Autodesk Inventor part; units mm, degrees
ref_plane "YZ Plane" through (0, 0, 0) normal (1, 0, 0) x (0, 1, 0)
ref_plane "XZ Plane" through (0, 0, 0) normal (0, 1, 0) x (-1, 0, 0)
ref_plane "XY Plane" through (0, 0, 0) normal (0, 0, 1) x (1, 0, 0)
sketch "スケッチ1" plane through (0, 0, 0) normal (0, 1, 0) x (-1, 0, 0)
  line L0 (75, 0) -> (105, -51.9615)
  line L1 (-75, 0) -> (-105, -51.9615)
  line L2 (0, -218.2384) -> (0, 36.3731)
  line L3 (147, 0) -> (-147, 0)
  line L4 (105, -51.9615) -> (30, -181.8653)
  line L5 (30, -181.8653) -> (-30, -181.8653)
  line L6 (-30, -181.8653) -> (-105, -51.9615)
  line L7 (75, 0) -> (-75, 0)
  line L8 (34, 0) -> (34, -24.3509)
  line L9 (34, -24.3509) -> (48.7058, -49.822)
  line L10 (48.7058, -49.822) -> (90, -25.9808)
  line L11 (45, 0) -> (45, -18) construction
  line L12 (45, -18) -> (34, -24.3509) construction
  line L13 (84.5, -87.4686) -> (63.4115, -75.2931)
  line L14 (63.4115, -75.2931) -> (48.7058, -49.822)
  line L15 (-34, 0) -> (-34, -24.3509)
  line L16 (-34, -24.3509) -> (-48.7058, -49.822)
  line L17 (-63.4115, -75.2931) -> (-48.7058, -49.822)
  line L18 (-84.5, -87.4686) -> (-63.4115, -75.2931)
  circle A0 centre (30, -32.75) radius 1.6
  circle A1 centre (-30, -32.75) radius 1.6
  line L19 (35.5295, -27) -> (-35.5295, -27)
  point P0 (0, 0)
  point P1 (0, 0)
  point P2 (0, -27)
  dimension "d1" = 150
  dimension "d2" = 60
  dimension "d3" = 60
  dimension "d6" = 60
  dimension "d30" = 60
  dimension "d31" = 18
  dimension "d32" = 30
  dimension "d33" = 41
  dimension "d34" = 3.2
  dimension "d35" = 30
  dimension "d36" = 32.75
  dimension "d37" = 27
extrude "プレート1" add sketch "スケッチ1" along normal blind 1.5 contours L14 L13 L4 L5 L2 L19 L9 | L2 L5 L6 L18 L17 L16 L19
sketch "スケッチ4" plane through (0, 1.5, 0) normal (0, 1, 0) x (1, 0, 0)
  circle A0 centre (30, 67.8013) radius 1.6
  circle A1 centre (45, 67.8013) radius 1.6
  line L0 (0, 218.2384) -> (0, -36.3731)
  circle A2 centre (-30, 67.8013) radius 1.6
  circle A3 centre (-45, 67.8013) radius 1.6
  line L1 (61.6173, 73.1025) -> (25, 73.1025)
  line L2 (25, 73.1025) -> (25, 62.5)
  line L3 (-61.6173, 73.1025) -> (-25, 73.1025)
  line L4 (-25, 73.1025) -> (-25, 62.5)
  line L5 (-25, 62.5) -> (25, 62.5)
  line L6 (-30, 73.1025) -> (30, 73.1025)
  line L7 (30, 73.1025) -> (30, 181.8653)
  line L8 (30, 181.8653) -> (-30, 181.8653)
  line L9 (-30, 181.8653) -> (-30, 73.1025)
  line L10 (-25, 62.5) -> (25, 62.5)
  line L11 (25, 62.5) -> (25, 73.1025)
  line L12 (25, 73.1025) -> (-25, 73.1025)
  line L13 (-25, 73.1025) -> (-25, 62.5)
  line L14 (30, 181.8653) -> (84.5, 87.4686)
  line L15 (76.75, 100.892) -> (30, 73.9008)
  line L16 (-30, 73.9008) -> (-76.75, 100.892)
  line L17 (-84.5, 87.4686) -> (-30, 181.8653)
  line L18 (84.5, 87.4686) -> (63.4115, 75.2931)
  line L19 (-63.4115, 75.2931) -> (-84.5, 87.4686)
  line L20 (-35.5295, 27) -> (-63.4115, 75.2931)
  line L21 (62.8673, 70.9375) -> (54.6673, 85.1403)
  arc A4 (54.6673, 85.1403) -> (44.275, 79.1403) centre (49.4712, 82.1403) ccw
  line L22 (44.275, 79.1403) -> (52.475, 64.9375)
  line L23 (52.475, 64.9375) -> (62.8673, 70.9375)
  line L24 (51.2321, 85.1903) -> (52.993, 82.1403)
  line L25 (52.993, 82.1403) -> (51.2321, 79.0903)
  line L26 (51.2321, 79.0903) -> (47.7102, 79.0903)
  line L27 (47.7102, 79.0903) -> (45.9493, 82.1403)
  line L28 (45.9493, 82.1403) -> (47.7102, 85.1903)
  line L29 (47.7102, 85.1903) -> (51.2321, 85.1903)
  point P0 (0, 0)
extrude "切り取り3" cut sketch "スケッチ4" against normal blind 1.5 contours A0 | A1 | L8 L7 L1 L6 L0 | L0 L6 L3 L9 L8 | L6 L2 L5 L0 | L0 L5 L4 L6 | L14 L15 A4 L7 | L9 L16 L17 | A4 L15 L29 L28 | L28 L29 L15 | A2 | A3
sketch "スケッチ5" plane through (0, 1.5, 0) normal (0, 1, 0) x (1, 0, 0)
  line L0 (-75, 44) -> (75, 44)
  circle A0 centre (-20, 41) radius 3
  circle A1 centre (20, 41) radius 3
  line L1 (-25, 62.5) -> (25, 62.5)
  line L2 (0, 62.5) -> (0, 27)
  line L3 (35.5295, 27) -> (-35.5295, 27)
  circle A2 centre (-20, 41) radius 1.6
  circle A3 centre (20, 41) radius 1.6
  circle A4 centre (0, 34) radius 1.6
  point P0 (0, 0)
  dimension "d41" = 6
  dimension "d42" = 6
  dimension "d43" = 40
  dimension "d44" = 3.2
  dimension "d45" = 3.2
  dimension "d46" = 3.2
  dimension "d47" = 7
extrude "切り取り4" cut sketch "スケッチ5" against normal blind 1.5 contours A4 L2 | L2 A4 | A2 | A3
sketch "スケッチ6" plane through (0, 1.5, 0) normal (0, 1, 0) x (1, 0, 0)
  ellipse E0 centre (-73.3666, 93.1522) end of major axis (-72.2841, 92.5272) minor radius 1.2133
  circle A0 centre (-48.4391, 79.9279) radius 1.6
  circle A1 centre (-73.3666, 93.1522) radius 1.6
  line L0 (0, 0) -> (0, 20.4537)
  circle A2 centre (48.4391, 79.9279) radius 1.6
  circle A3 centre (73.3666, 93.1522) radius 1.6
  circle A4 centre (-48.4391, 79.9279) radius 1.35
  dimension "d51" = 3.2
  dimension "d52" = 3.2
extrude "切り取り5" cut sketch "スケッチ6" against normal blind 1.5 contours E0 | A0 | A1 | A2 | A3 | A4
equation "\"d3\" = d2"
equation "\"d38\" = Thickness"
equation "\"d41\" = d42"
equation "\"d48\" = Thickness"
equation "\"d53\" = Thickness"
equation "\"d16\" = Thickness"
equation "\"BendRadius\" = Thickness"
equation "\"BendReliefWidth\" = Thickness"
equation "\"BendReliefDepth\" = 0.5 * Thickness"
equation "\"CornerReliefSize\" = 4 * Thickness"
equation "\"MinimumRemnant\" = 2 * Thickness"
equation "\"TransitionRadius\" = BendRadius"
equation "\"JacobiRadiusSize\" = BendRadius"
equation "\"GapSize\" = Thickness"
properties part number "upper_plate" material "アルミニウム 6061"
Input: part model. Units: mm. Frame: model coordinates. Give positions to 0.01 mm unless a question says otherwise; leave off trailing zeros. Write each loop counter-clockwise with the first axis right and the second up, starting at its lowest first coordinate (ties: lowest second). Pieces come first, ordered by that corner, then holes.
Q1. Section B-B, the plane z = -64.5. Output: boundary loops of the cut face in (x, y), plus the area to 3 significant figures.
Q2. Section A-A, the plane x = 20. Output: boundary loops of the cut face in (y, z), plus the area to 4 significant figures.
Q3. Material intervals for probe 1 along X at (y, z) = (0.65, -79); probe 2 along X at (y, z) = (0.7, -41); probe 3 along Z at (x, y) = (0, 1.15), sorted ascending.
Q4. First-contact query: P1, Ø0.8, axis at y = 0.5, z = -68.5, coming from the +X side; P2, Ø0.6, axis at y = 1, z = -73.5, coming from the +X side. Flat tips, straight axial feed; report the tip coordinate or a pass-through.
Q5. Section D-D, the plane y = 0.3. State how many separate pieces and enclosed holes the cut face has, plus the area to 3 significant figures.
Q6. Section C-C, the plane z = -41. Output: boundary loops of the cut face in (x, y), plus the area to 3 significant figures.
Q7. Pull-direction query (X, two-part tool) for faces 1 (the face through (74.103, 0.74, -81.466)), 2 (the face through (53.702, 0.76, -87.585)), 3 (the face through (-80.679, 0.74, -94.086)), 4 (the face through (49.18, 0.76, -78.51)); classes: pulls with the +X half, pulls with the -X half, needs draft (parallel to the pull), parting line crosses it, or undercut.
Filled in:
1. outline: (-57.18, 0) - (-25, 0) - (-25, 1.5) - (-57.18, 1.5) - close; (25, 0) - (57.18, 0) - (57.18, 1.5) - (25, 1.5) - close
1. area: 96.5 mm2
2. outline: (0, -62.5) - (1.5, -62.5) - (1.5, -42.6) - (0, -42.6) - close; (0, -39.4) - (1.5, -39.4) - (1.5, -27) - (0, -27) - close
2. area: 48.45 mm2
3. probe 1: x = -69.83 to -49.74, -47.14 to -38.83, 38.83 to 47.14, 49.74 to 69.83
3. probe 2: x = -43.61 to -21.6, -18.4 to 18.4, 21.6 to 43.61
3. probe 3: z = -62.5 to -35.6, -32.4 to -27
4. P1: stops at x = 59.72
4. P2: stops at x = 62.55
5. separate pieces: 1
5. enclosed holes: 13
5. area: 5,180 mm2
6. outline: (-43.61, 0) - (-21.6, 0) - (-21.6, 1.5) - (-43.61, 1.5) - close; (-18.4, 0) - (18.4, 0) - (18.4, 1.5) - (-18.4, 1.5) - close; (21.6, 0) - (43.61, 0) - (43.61, 1.5) - (21.6, 1.5) - close
6. area: 121 mm2
7. face 1: pulls with the +X half
7. face 2: undercut
7. face 3: pulls with the -X half
7. face 4: undercut
